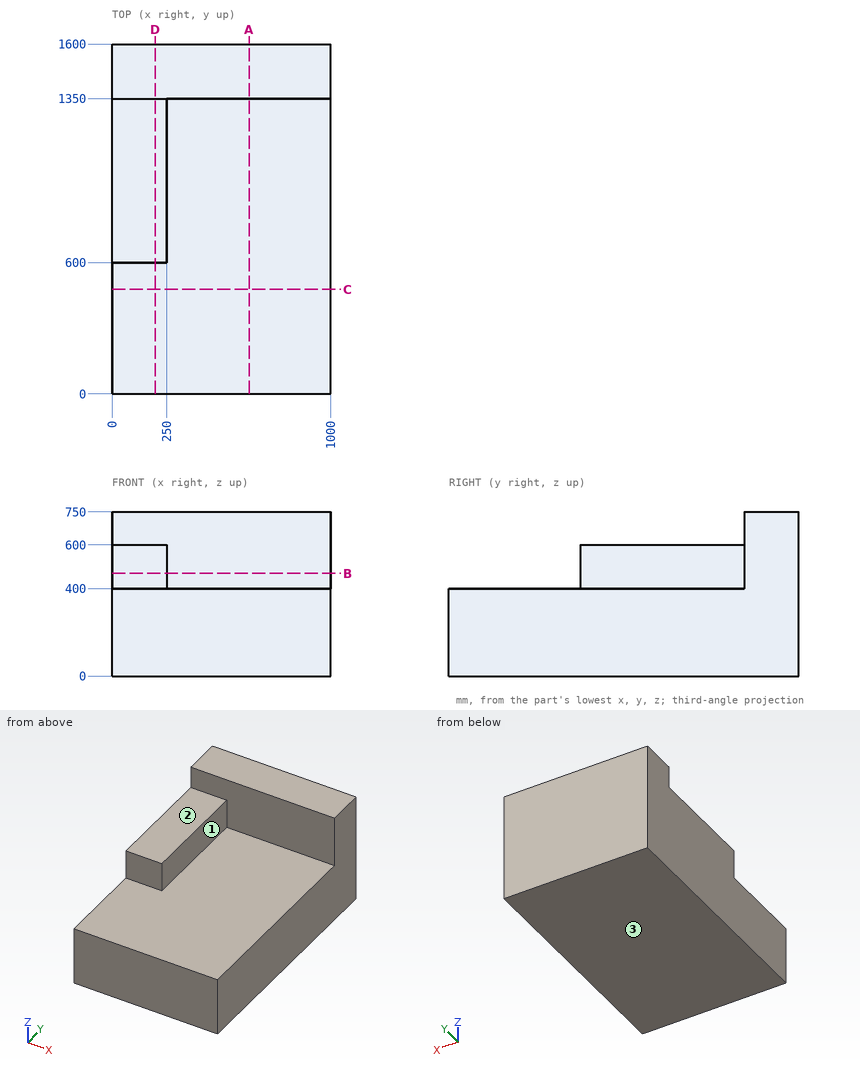
Design review of the part shown in the three views and the two pictorial views. Dimensions are in mm from the part's minimum x, y and z. A direction names the side the tool comes from. Give positions to 0.01 mm unless a question says otherwise; leave off trailing zeros. Write each loop counter-clockwise with the first axis right and the second up, starting at its lowest first coordinate (ties: lowest second). Pieces come first, ordered by that corner, then holes.
(1) Wall thickness on line 1 along Y through (x, z) = (456, 639.5); line 2 along Z through (x, y) = (822, 303); line 3 along Z through (x, y) = (212.5, 993.5): over which ranges is each line inside the solid? List them lowest first.
Checked values:
line 1: y = 1350 to 1600
line 2: z = 0 to 400
line 3: z = 0 to 600
(2) Clearance check with flat-ended pins moving along their axes: pin 1 Ø1.5 at (x, y) = (320.5, 1270.5) entering from +Z; pin 2 Ø1.5 at (x, z) = (150.5, 494.5) entering from -Y. State where each tip first meets the part, or that it passes through.
Checked values:
pin 1: stops at z = 400
pin 2: stops at y = 600
(3) Add section C-C (y = 478.5). Give the boundary of the cut face in (x, z).
Checked values:
outline: (0, 0) - (1000, 0) - (1000, 400) - (0, 400) - close
(4) Add section D-D (x = 196). Give the boundary of the cut face in (y, z), and give its area (4 significant figures).
Checked values:
outline: (0, 0) - (1600, 0) - (1600, 750) - (1350, 750) - (1350, 600) - (600, 600) - (600, 400) - (0, 400) - close
area: 877,500 mm2
(5) Add section B-B (z = 469.5). Give the boundary of the cut face in (x, y).
Checked values:
outline: (0, 600) - (250, 600) - (250, 1350) - (1000, 1350) - (1000, 1600) - (0, 1600) - close
(6) Add section A-A (x = 626.5). Give the boundary of the cut face in (y, z), and give its area (4 significant figures).
Checked values:
outline: (0, 0) - (1600, 0) - (1600, 750) - (1350, 750) - (1350, 400) - (0, 400) - close
area: 727,500 mm2
(7) Tool access review of the marked faces 1, 2 and 3: name each direction out of +Z, -Z, +X, -X, +Y, -Y from which nothing blocks a thin tool from reaching the whole face with its end or side.
Checked values:
face 1: +Z, +X, -Y
face 2: +Z, +X, -X, -Y
face 3: -Z, +X, -X, +Y, -Y
